```python
from build123d import *

# Parameters (mm, degrees)
SKETCH_1_W           = 120
SKETCH_1_H           = 120
EXTRUDE_1_DEPTH      = 3
SKETCH_2_W           = 123
SKETCH_2_H           = 128
EXTRUDE_2_DEPTH      = 5
SKETCH_4_R           = 22.5
CUT_EXTRUDE_2_DEPTH  = 90.119302062
SKETCH_5_W           = 15.3
SKETCH_5_H           = 19
SKETCH_5_W_2         = 12.6
SKETCH_5_H_2         = 16
CUT_EXTRUDE_3_DEPTH  = 3
SKETCH_3_R           = 1.7
CUT_EXTRUDE_5_DEPTH  = 90.119302062
SKETCH_15_R          = 1.35
CUT_EXTRUDE_7_DEPTH  = 90.119302062
SKETCH_20_R          = 2.6
SKETCH_20_R_2        = 2.1
CUT_EXTRUDE_14_DEPTH = 90.119302062
SKETCH_21_R          = 5.5
SKETCH_21_R_2        = 4.6
CUT_EXTRUDE_15_DEPTH = 1
SKETCH_23_W          = 1
SKETCH_23_H          = 5
EXTRUDE_5_DEPTH      = 123
FILLET_1_R           = 0.5
SKETCH_25_R          = 0.5
CUT_EXTRUDE_17_DEPTH = 3
FILLET_2_R           = 1
CHAMFER_1_SIZE       = 0.2


with BuildPart() as part:
    # 草图1 → 凸台-拉伸1 (new body)
    with BuildSketch(Plane(origin=(0, 0, 0), x_dir=(1, 0, 0), z_dir=(0, 1, 0))):
        Rectangle(SKETCH_1_W, SKETCH_1_H)
    extrude(amount=EXTRUDE_1_DEPTH)

    # 草图2 → 凸台-拉伸2 (add)
    with BuildSketch(Plane.XZ):
        Rectangle(SKETCH_2_W, SKETCH_2_H)
    extrude(amount=EXTRUDE_2_DEPTH)

    # 草图4 → 切除-拉伸2 (cut, through all)
    with BuildSketch(Plane(origin=(0, 3, 0), x_dir=(1, 0, 0), z_dir=(0, 1, 0))):
        with Locations(Location((0, 0, 0), (0, 0, 270))):
            Circle(SKETCH_4_R)
    extrude(amount=-CUT_EXTRUDE_2_DEPTH, mode=Mode.SUBTRACT)

    # 草图5 → 切除-拉伸3 (cut)
    with BuildSketch(Plane(origin=(0, 3, 0), x_dir=(1, 0, 0), z_dir=(0, 1, 0))):
        with Locations((-53.85, 54.5)):
            Rectangle(SKETCH_5_W, SKETCH_5_H)
        with Locations((35.4, 56)):
            Rectangle(SKETCH_5_W_2, SKETCH_5_H_2)
        with Locations((53.85, 54.5)):
            Rectangle(SKETCH_5_W, SKETCH_5_H)
        with Locations((-35.4, 56)):
            Rectangle(SKETCH_5_W_2, SKETCH_5_H_2)
        with Locations((-53.85, -54.5)):
            Rectangle(SKETCH_5_W, SKETCH_5_H)
        with Locations((53.85, -54.5)):
            Rectangle(SKETCH_5_W, SKETCH_5_H)
    extrude(amount=-CUT_EXTRUDE_3_DEPTH, mode=Mode.SUBTRACT)

    # 草图3 → 切除-拉伸5 (cut, through all)
    with BuildSketch(Plane(origin=(0, 3, 0), x_dir=(1, 0, 0), z_dir=(0, 1, 0))):
        with Locations(Location((0, 51, 0), (0, 0, 270))):
            Circle(SKETCH_3_R)
        with Locations(Location((25.5, 44.167295593, 0), (0, 0, 270))):
            Circle(SKETCH_3_R)
        with Locations(Location((44.167295593, 25.5, 0), (0, 0, 270))):
            Circle(SKETCH_3_R)
        with Locations(Location((51, 0, 0), (0, 0, 270))):
            Circle(SKETCH_3_R)
        with Locations(Location((44.167295593, -25.5, 0), (0, 0, 270))):
            Circle(SKETCH_3_R)
        with Locations(Location((25.5, -44.167295593, 0), (0, 0, 270))):
            Circle(SKETCH_3_R)
        with Locations(Location((0, -51, 0), (0, 0, 270))):
            Circle(SKETCH_3_R)
        with Locations(Location((-25.5, -44.167295593, 0), (0, 0, 270))):
            Circle(SKETCH_3_R)
        with Locations(Location((-44.167295593, -25.5, 0), (0, 0, 270))):
            Circle(SKETCH_3_R)
        with Locations(Location((-51, 0, 0), (0, 0, 270))):
            Circle(SKETCH_3_R)
        with Locations(Location((-44.167295593, 25.5, 0), (0, 0, 270))):
            Circle(SKETCH_3_R)
        with Locations(Location((-25.5, 44.167295593, 0), (0, 0, 270))):
            Circle(SKETCH_3_R)
    extrude(amount=-CUT_EXTRUDE_5_DEPTH, mode=Mode.SUBTRACT)

    # 草图15 → 切除-拉伸7 (cut, through all)
    with BuildSketch(Plane(origin=(0, 3, 0), x_dir=(1, 0, 0), z_dir=(0, 1, 0))):
        with Locations(Location((0, -33, 0), (0, 0, 270))):
            Circle(SKETCH_15_R)
        with Locations(Location((0, -43, 0), (0, 0, 270))):
            Circle(SKETCH_15_R)
        with Locations(Location((-33, 0, 0), (0, 0, 270))):
            Circle(SKETCH_15_R)
        with Locations(Location((-43, 0, 0), (0, 0, 270))):
            Circle(SKETCH_15_R)
    extrude(amount=-CUT_EXTRUDE_7_DEPTH, mode=Mode.SUBTRACT)

    # 草图20 → 切除-拉伸14 (cut, through all)
    with BuildSketch(Plane(origin=(0, 3, 0), x_dir=(1, 0, 0), z_dir=(0, 1, 0))):
        with Locations(Location((-53.85, 52.5, 0), (0, 0, 270))):
            Circle(SKETCH_20_R)
        with Locations(Location((-53.85, -52.5, 0), (0, 0, 270))):
            Circle(SKETCH_20_R)
        with Locations(Location((53.85, -52.5, 0), (0, 0, 270))):
            Circle(SKETCH_20_R)
        with Locations(Location((53.85, 52.5, 0), (0, 0, 270))):
            Circle(SKETCH_20_R)
        with Locations(Location((-35.4, 54, 0), (0, 0, 270))):
            Circle(SKETCH_20_R_2)
        with Locations(Location((35.4, 54, 0), (0, 0, 270))):
            Circle(SKETCH_20_R_2)
    extrude(amount=-CUT_EXTRUDE_14_DEPTH, mode=Mode.SUBTRACT)

    # 草图21 → 切除-拉伸15 (cut)
    with BuildSketch(Plane.XZ.offset(5)):
        with Locations(Location((53.85, -52.5, 0), (0, 0, 270))):
            Circle(SKETCH_21_R)
        with Locations(Location((35.4, -54, 0), (0, 0, 270))):
            Circle(SKETCH_21_R_2)
        with Locations(Location((-35.4, -54, 0), (0, 0, 270))):
            Circle(SKETCH_21_R_2)
        with Locations(Location((-53.85, -52.5, 0), (0, 0, 270))):
            Circle(SKETCH_21_R)
        with Locations(Location((-53.85, 52.5, 0), (0, 0, 270))):
            Circle(SKETCH_21_R)
        with Locations(Location((53.85, 52.5, 0), (0, 0, 270))):
            Circle(SKETCH_21_R)
    extrude(amount=-CUT_EXTRUDE_15_DEPTH, mode=Mode.SUBTRACT)

    # 草图23 → 凸台-拉伸5 (add)
    with BuildSketch(Plane.ZY.offset(61.5)):
        with Locations((-64.5, -2.5)):
            Rectangle(SKETCH_23_W, SKETCH_23_H)
        with Locations((64.5, -2.5)):
            Rectangle(SKETCH_23_W, SKETCH_23_H)
    extrude(amount=-EXTRUDE_5_DEPTH)

    # 圆角1
    fillet_1_edges = [part.edges().sort_by_distance(p)[0] for p in [
        (46.2, 1.5, 60),
        (60, 1.5, 45),
        (-46.2, 1.5, -60),
        (-60, 1.5, -45),
        (-60, 1.5, 45),
        (-46.2, 1.5, 60),
        (41.7, 1.5, -60),
        (29.1, 1.5, -60),
        (-29.1, 1.5, -60),
        (-41.7, 1.5, -60),
        (60, 1.5, -45),
        (46.2, 1.5, -60),
    ]]
    fillet(fillet_1_edges, radius=FILLET_1_R)

    # 草图25 → 切除-拉伸17 (cut)
    with BuildSketch(Plane(origin=(0, 3, 0), x_dir=(1, 0, 0), z_dir=(0, 1, 0))):
        with Locations((-46.7, 45)):
            Circle(SKETCH_25_R)
        with Locations((-41.2, 48)):
            Circle(SKETCH_25_R)
        with Locations((41.2, 48)):
            Circle(SKETCH_25_R)
        with Locations((46.7, 45)):
            Circle(SKETCH_25_R)
        with Locations((-46.7, -45)):
            Circle(SKETCH_25_R)
        with Locations((46.7, -45)):
            Circle(SKETCH_25_R)
        with Locations((-29.6, 48)):
            Circle(SKETCH_25_R)
        with Locations((29.6, 48)):
            Circle(SKETCH_25_R)
    extrude(amount=-CUT_EXTRUDE_17_DEPTH, mode=Mode.SUBTRACT)

    # 圆角2
    fillet_2_edges = [part.edges().sort_by_distance(p)[0] for p in [
        (30.1, 1.5, -48),
        (40.7, 1.5, -48),
        (-30.1, 1.5, -48),
        (-40.7, 1.5, -48),
        (47.2, 1.5, 45),
        (-47.2, 1.5, -45),
        (47.2, 1.5, -45),
        (-47.2, 1.5, 45),
    ]]
    fillet(fillet_2_edges, radius=FILLET_2_R)

    # 倒角1
    chamfer_1_edges = [part.edges().sort_by_distance(p)[0] for p in [
        (61.5, -5, 0),
        (-61.5, -5, 0),
        (0, -5, -65),
        (0, -5, 65),
    ]]
    chamfer(chamfer_1_edges, length=CHAMFER_1_SIZE)


solid = part.part
```
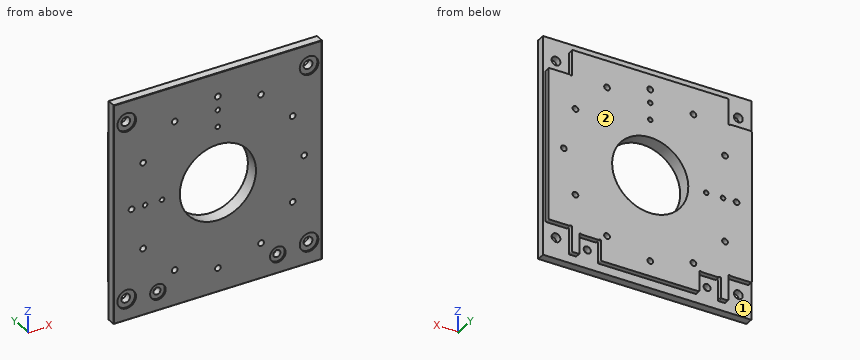
The listing builds one solid part. Answer for the finished solid, in the listing's coordinates (mm). Face numbers are marked on the shaded views. A direction names the side the tool comes from. Coordinates: 2 decimals unless noted, no trailing zeros. Write each loop counter-clockwise with the first axis right and the second up, starting at its lowest first coordinate (ties: lowest second). Pieces come first, ordered by that corner, then holes. Notation, with made-up numbers: (-2, 73) - (40, 73) arc R8 cw to (40, 80) - close; hole circle Ø7 at (-29.75, 75.5). An arc over 180 degrees is marked (long way). Return JSON: item names as keys, results as strings. Group by question number.
1. Given pin 1 (2.5 mm diameter, centred on y = 1.5, z = -55, fed in from +X); pin 2 (0.9 mm diameter, centred on x = -11, y = 1.5, fed in from -Z); pin 3 (5.5 mm diameter, centred on x = -35.4, z = -54, fed in from +Y); pin 4 (2 mm diameter, centred on x = 44.17, z = -25.5, fed in from -Y), each flat-ended and moving along its own axis, determine where each tip first touches the part or whether it passes through.
2. Straight lines are drawn through the part: L1, parallel to X at y = -0.25, z = 0; L2, parallel to Z at x = -52, y = 1.5; L3, parallel to X at y = 0.5, z = 51. For each, find the intervals that lie inside material, in ascending order.
3. A cutting plane is placed at D-D, the plane y = -2. Give the number of separate pieces and of enclosed holes in the cut face, plus the area to 3 significant figures.
4. A cutting plane is placed at A-A, the plane x = 35.4. Determine the outline of the cut face in (y, z), plus the area to 3 significant figures.
5. Which of the six approach directions +Z, -Z, +X, -X, +Y, -Y give full straight-line access (tool end or side, diameter ignored) to the marked faces 1 and 2?
6. A cutting plane is placed at C-C, the plane z = -11. Determine the outline of the cut face in (x, y), plus the area to 3 significant figures.
7. A cutting plane is placed at B-B, the plane z = 25.5. Determine the outline of the cut face in (x, y), plus the area to 3 significant figures.
Ans:
{
 "1": {"pin 1": "x = 46.2", "pin 2": "z = -60", "pin 3": "y = 0", "pin 4": "through"},
 "2": {"L1": "-61.5 to -52.7, -49.3 to -44.35, -41.65 to -34.35, -31.65 to -22.5, 22.5 to 49.3, 52.7 to 61.5", "L2": "-45 to -1.37, 1.37 to 45", "L3": "-46.2 to -1.7, 1.7 to 46.2"},
 "3": {"separate pieces": "1", "enclosed holes": "23", "area": "14,200 mm²"},
 "4": {"outline": "(-5, -64.8) - (-4.8, -65) - (0, -65) - (0, -56.1) - (-4, -56.1) - (-4, -58.6) - (-5, -58.6) - close; (-5, -49.4) - (-4, -49.4) - (-4, -51.9) - (0, -51.9) - (0, -48) - (3, -48) - (3, 60) - (0, 60) - (0, 65) - (-4.8, 65) - (-5, 64.8) - close", "area": "948 mm²"},
 "5": {"face 1": "+Y", "face 2": "+Z, -Z, +X, -X, +Y"},
 "6": {"outline": "(-61.5, -4.8) - (-61.3, -5) - (-19.63, -5) - (-19.63, 3) - (-60, 3) - (-60, 0) - (-61.5, 0) - close; (19.63, -5) - (61.3, -5) - (61.5, -4.8) - (61.5, 0) - (60, 0) - (60, 3) - (19.63, 3) - close", "area": "661 mm²"},
 "7": {"outline": "(-61.5, -4.8) - (-61.3, -5) - (-45.87, -5) - (-45.87, 3) - (-60, 3) - (-60, 0) - (-61.5, 0) - close; (-42.47, -5) - (42.47, -5) - (42.47, 3) - (-42.47, 3) - close; (45.87, -5) - (61.3, -5) - (61.5, -4.8) - (61.5, 0) - (60, 0) - (60, 3) - (45.87, 3) - close", "area": "921 mm²"}
}
